```python
from build123d import *

# Parameters (mm, degrees)
ESQUISSE2_W                  = 4
ESQUISSE2_H                  = 7.3
ENL_V_MAT_EXTRU_1_DEPTH      = 31.221184623
ENL_V_MAT_EXTRU_2_DEPTH      = 30.306014741
R_P_TITION_CIRCULAIRE1_COUNT = 9


with BuildPart() as part:
    # Esquisse1 → R_volution1 (revolve)
    with BuildSketch(Plane(origin=(0, 0, 0), x_dir=(0, 0, -1), z_dir=(1, 0, 0)), mode=Mode.PRIVATE) as r_volution1_sk:
        Polygon((-5.8, 20.4), (-6.6, 17.5), (-6.6, 10.5), (-9, 10.5), (-9, 5.5), (0, 5.5), (0, 10.5), (-3.7, 10.5), (-3.7, 17.5), (-4.5, 20.4), align=None)
    revolve(r_volution1_sk.sketch.rotate(Axis((0, 0, 0), (0, 0, 1)), 90), axis=Axis((0, 0, 0), (0, 0, 1)))

    # Esquisse2 → Enl_v. mat.-Extru.1 (cut, through all)
    with BuildSketch(Plane.XY):
        with Locations((0, 3.65)):
            Rectangle(ESQUISSE2_W, ESQUISSE2_H)
    extrude(amount=ENL_V_MAT_EXTRU_1_DEPTH, mode=Mode.SUBTRACT)

    # Esquisse4 → Enl_v. mat.-Extru.2 (cut, symmetric)
    with BuildSketch(Plane.XY.offset(5.15)):
        with BuildLine():
            ThreePointArc((-3.488153141, 16.878433832), (0, 14.691157941), (3.488153141, 16.878433832))
            ThreePointArc((3.488153141, 16.878433832), (4.416914632, 18.359445416), (5.645191484, 19.603362291))
            ThreePointArc((5.645191484, 19.603362291), (0, 20.4), (-5.645191484, 19.603362291))
            ThreePointArc((-5.645191484, 19.603362291), (-4.416914632, 18.359445416), (-3.488153141, 16.878433832))
        make_face()
    enl_v_mat_extru_2 = extrude(amount=ENL_V_MAT_EXTRU_2_DEPTH, both=True, mode=Mode.SUBTRACT)

    # R_p_tition circulaire1: Enl_v. mat.-Extru.2 ×9 about axis
    r_p_tition_circulaire1_axis = Axis((0, 0, 0), (0, 0, 1))
    for i in range(1, R_P_TITION_CIRCULAIRE1_COUNT):
        add(enl_v_mat_extru_2.rotate(r_p_tition_circulaire1_axis, i * 360 / R_P_TITION_CIRCULAIRE1_COUNT), mode=Mode.SUBTRACT)


solid = part.part
```
Work out the finished part from the listing and answer in its coordinate system (mm). A direction names the side the tool comes from. Round coordinates to 2 decimals unless told otherwise and drop trailing zeros. Write each loop counter-clockwise with the first axis right and the second up, starting at its lowest first coordinate (ties: lowest second). Pieces come first, ordered by that corner, then holes.
1) Flat-ended cylindrical pins translate along their axes: P1, Ø17.5, axis at x = -5, y = -2, coming from the -Z side; P2, Ø4, axis at x = -13.5, y = -9.5, coming from the +Z side; P3, Ø2, axis at y = 7, z = 1.5, coming from the +X side; P4, Ø0.7, axis at y = 6, z = 5, coming from the -X side. Find the tip coordinate at first contact, or state that the pin passes through.
2) A cutting plane is placed at C-C on z = 7.75. Determine the outline of the cut face in (x, y), and give its area (3 significant figures).
3) A cutting plane is placed at A-A on x = 0. Determine the outline of the cut face in (y, z).
4) Determine the mould class of faces 1 (the face through (-10.083, -15.516, 5.17)), 2 (the face through (-17.657, 10.217, 5.159)), 3 (the face through (-4.2, 18.07, 5.17)), 4 (the face through (18.318, -3.267, 6.294)) for opening direction X: pulls with the +X half, pulls with the -X half, needs draft (parallel to the pull), parting line crosses it, or undercut.
5) A cutting plane is placed at B-B on y = 1. Determine the outline of the cut face in (x, z).
6) Which of the six approach directions +Z, -Z, +X, -X, +Y, -Y give full straight-line access (tool end or side, diameter ignored) to faces 5 (the face through (-10, -3.2, 7.8)), 6 (the face through (-13.55, -12.67, 5.17)), 7 (the face through (4.17, 18.03, 5.17))?
7) Consider probe 1 along Y at (x, z) = (0, 3.5); probe 2 along Y at (x, z) = (0, 4.75); probe 3 along Z at (x, y) = (-12, -3). Determine where each line is inside the solid, lowest interval first.
Entries:
1. P1: stops at z = 0
1. P2: stops at z = 6.6
1. P3: stops at x = 8.62
1. P4: stops at x = -15.99
2. outline: circle Ø21 at (0, 0); hole (-2, 5.12) arc R5.5 ccw (long way) to (2, 5.12) - (2, 7.3) - (-2, 7.3) - close
2. area: 244 mm2
3. outline: (-20.4, 4.5) - (-17.5, 3.7) - (-10.5, 3.7) - (-10.5, 0) - (-5.5, 0) - (-5.5, 9) - (-10.5, 9) - (-10.5, 6.6) - (-17.5, 6.6) - (-20.4, 5.8) - close; (7.3, 0) - (10.5, 0) - (10.5, 3.7) - (14.69, 3.7) - (14.69, 6.6) - (10.5, 6.6) - (10.5, 9) - (7.3, 9) - close
4. face 1: undercut
4. face 2: pulls with the -X half
4. face 3: undercut
4. face 4: pulls with the +X half
5. outline: (-15.11, 3.7) - (-10.45, 3.7) - (-10.45, 0) - (-5.41, 0) - (-5.41, 9) - (-10.45, 9) - (-10.45, 6.6) - (-15.11, 6.6) - close; (5.41, 0) - (10.45, 0) - (10.45, 3.7) - (15.11, 3.7) - (15.11, 6.6) - (10.45, 6.6) - (10.45, 9) - (5.41, 9) - close
6. face 5: +Z
6. face 6: +Z, -Z, -X
6. face 7: +Z, -Z, +Y
7. probe 1: y = -10.5 to -5.5, 7.3 to 10.5
7. probe 2: y = -20.4 to -5.5, 7.3 to 14.69
7. probe 3: z = 3.7 to 6.6
